from build123d import *

# Parameters (mm, degrees)
SKETCH_1_W               = 85
SKETCH_1_H               = 300
EXTRUDE_1_DEPTH          = 820
SKETCH_2_W               = 77.5
SKETCH_2_H               = 273
CUT_EXTRUDE_1_DEPTH      = 878.282736636
SKETCH_5_W               = 50
SKETCH_5_H               = 140
EXTRUDE_3_DEPTH          = 11
SKETCH_6_W               = 80
SKETCH_6_H               = 158
EXTRUDE_4_DEPTH          = 18
MIRROR_4_COPY_1_SKETCH_W = 50
MIRROR_4_COPY_1_SKETCH_H = 140
MIRROR_4_COPY_1_DEPTH    = 11
MIRROR_4_COPY_2_SKETCH_W = 80
MIRROR_4_COPY_2_SKETCH_H = 158
MIRROR_4_COPY_2_DEPTH    = 18


with BuildPart() as part:
    # 草图1 → 凸台-拉伸1 (new body)
    with BuildSketch(Plane.XY):
        with Locations((42.5, 150)):
            Rectangle(SKETCH_1_W, SKETCH_1_H)
    extrude(amount=EXTRUDE_1_DEPTH)

    # 草图2 → 切除-拉伸1 (cut, through all)
    with BuildSketch(Plane.XY.offset(820)):
        with Locations((46.25, 150)):
            Rectangle(SKETCH_2_W, SKETCH_2_H)
    extrude(amount=-CUT_EXTRUDE_1_DEPTH, mode=Mode.SUBTRACT)

    # 草图5 → 凸台-拉伸3 (add)
    with BuildSketch(Plane.XZ.offset(-286.5)):
        with Locations((46.25, 70)):
            Rectangle(SKETCH_5_W, SKETCH_5_H)
    extrude_3 = extrude(amount=EXTRUDE_3_DEPTH)

    # 草图6 → 凸台-拉伸4 (add)
    with BuildSketch(Plane(origin=(0, 300, 0), x_dir=(1, 0, 0), z_dir=(0, 1, 0))):
        with Locations((42.5, -61)):
            Rectangle(SKETCH_6_W, SKETCH_6_H)
    extrude_4 = extrude(amount=EXTRUDE_4_DEPTH)

    # 镜向3: 凸台-拉伸3, 凸台-拉伸4 across plane
    add(extrude_3.mirror(Plane(origin=(0, 150, 0), x_dir=(0, 0, 1), z_dir=(0, -1, 0))))
    add(extrude_4.mirror(Plane(origin=(0, 150, 0), x_dir=(0, 0, 1), z_dir=(0, -1, 0))))

    # 镜向4: 凸台-拉伸3, 凸台-拉伸4 across plane
    add(extrude_3.mirror(Plane(origin=(0, 0, 410), x_dir=(1, 0, 0), z_dir=(0, 0, -1))))
    add(extrude_4.mirror(Plane(origin=(0, 0, 410), x_dir=(1, 0, 0), z_dir=(0, 0, -1))))

    # 镜向4 copy 1 sketch → 镜向4 copy 1 (add)
    with BuildSketch(Plane(origin=(0, 13.5, 820), x_dir=(1, 0, 0), z_dir=(0, 1, 0))):
        with Locations((46.25, 70)):
            Rectangle(MIRROR_4_COPY_1_SKETCH_W, MIRROR_4_COPY_1_SKETCH_H)
    extrude(amount=MIRROR_4_COPY_1_DEPTH)

    # 镜向4 copy 2 sketch → 镜向4 copy 2 (add)
    with BuildSketch(Plane(origin=(0, 0, 820), x_dir=(1, 0, 0), z_dir=(0, -1, 0))):
        with Locations((42.5, -61)):
            Rectangle(MIRROR_4_COPY_2_SKETCH_W, MIRROR_4_COPY_2_SKETCH_H)
    extrude(amount=MIRROR_4_COPY_2_DEPTH)


solid = part.part
Build history of the part. All positions in model axes, mm. A direction names the side the tool comes from. Coordinates: 2 decimals unless noted, no trailing zeros. Order: outer loops, then holes, each group sorted by start corner. A loop starts at its lowest first (then second) coordinate and runs counter-clockwise, first axis right, second up. Notation, with made-up numbers: (88, -39.5) - (118, -39.5) arc R12 ccw to (118, -33.5) - close; hole circle Ø7 at (-24, -22). An arc over 180 degrees is marked (long way). Put each result on its own line as item: value.
1. Pull direction Y, two halves, no side cores. Call faces 6 (the face through (2.5, 309, 758)), 7 (the face through (42, -18, 760)), 8 (the face through (42, 300, 829)): pulls with the +Y half, pulls with the -Y half, needs draft (parallel to the pull), parting line crosses it, or undercut.
Answer sheet:
face 6: needs draft
face 7: pulls with the -Y half
face 8: undercut
2. Probe line 1 along Y through (x, z) = (25, 517); line 2 along Y through (x, z) = (73, 35); line 3 along Z through (x, y) = (47, 304.5). List the from-to ranges inside material, lowest first. Write a range as [from, to].
Answer sheet:
line 1: y = [0, 13.5], [286.5, 300]
line 2: y = [-18, 13.5], [286.5, 318]
line 3: z = [-18, 140], [680, 838]
3. Saw through at B-B (z = 41). Write the cut outline in (x, y).
Answer sheet:
outline: (0, 0) - (2.5, 0) - (2.5, -18) - (82.5, -18) - (82.5, 0) - (85, 0) - (85, 13.5) - (71.25, 13.5) - (71.25, 24.5) - (21.25, 24.5) - (21.25, 13.5) - (7.5, 13.5) - (7.5, 286.5) - (21.25, 286.5) - (21.25, 275.5) - (71.25, 275.5) - (71.25, 286.5) - (85, 286.5) - (85, 300) - (82.5, 300) - (82.5, 318) - (2.5, 318) - (2.5, 300) - (0, 300) - close
4. Saw through at D-D (z = 337.5). Write the cut outline in (x, y).
Answer sheet:
outline: (0, 0) - (85, 0) - (85, 13.5) - (7.5, 13.5) - (7.5, 286.5) - (85, 286.5) - (85, 300) - (0, 300) - close
5. Drop flat-ended pins along their axis: P1, Ø3.5, axis at y = 282, z = 39.5, coming from the +X side; P2, Ø8, axis at x = 73.5, y = 25.5, coming from the +Z side; P3, Ø3, axis at x = 68.5, z = 427.5, coming from the +Y side. Give the stop position or say it passes through.
Answer sheet:
P1: stops at x = 71.25
P2: stops at z = 820
P3: stops at y = 300
6. Tool access for faces 1 (the face through (82.5, -9, 758)), 2 (the face through (5, 151, 0)), 3 (the face through (42, 309, 680)), 4 (the face through (46, 275.5, 749)), 5 (the face through (42, -9, 140)): list every direction of +Z, -Z, +X, -X, +Y, -Y with a clear straight run to the whole face (end or side of a thin tool).
Answer sheet:
face 1: +Z, -Z, +X, -Y
face 2: -Z, +X, -X
face 3: +X, -X, +Y
face 4: +Z, -Z, +X
face 5: +X, -X, -Y
7. Saw through at C-C (y = 219.5). Write the cut outline in (x, z), and give its area (3 significant figures).
Answer sheet:
outline: (0, 0) - (7.5, 0) - (7.5, 820) - (0, 820) - close
area: 6,150 mm^2
